Input: dimensioned drawing with shaded views. Units: mm. Origin: part minimum x, y, z. A direction names the side the tool comes from. Round coordinates to 2 decimals unless told otherwise and drop trailing zeros. Loops run counter-clockwise (first coordinate to the right, second up) from the corner with the lowest first, then second, coordinate; pieces in that order, holes last. Notation, with made-up numbers: (-16, 38.5) - (16, 38.5) arc R8 cw to (16, 43.5) - close; hole circle Ø6 at (31.5, 9.25). An arc over 180 degrees is marked (long way). One line per question, with ' | ' between items. Start each with the question number.
Item 1: Material intervals for line 1 along Z through (x, y) = (4.25, 13.75); line 2 along Z through (x, y) = (3, 7.25); line 3 along Y through (x, z) = (12.75, 0.6), sorted ascending.
Item 2: Section C-C, the plane y = 14.75. Return loops of the section in (x, z).
Item 3: First-contact query: pin 1 (1.4 mm diameter, centred on x = 11, z = 1, fed in from +Y); pin 2 (3 mm diameter, centred on y = 4.5, z = 4, fed in from +X); pin 3 (2.5 mm diameter, centred on x = 3.5, y = 12, fed in from -Z); pin 4 (1.4 mm diameter, centred on y = 11, z = 0.5, fed in from +X). Flat tips, straight axial feed; report the tip coordinate or a pass-through.
Item 4: Section B-B, the plane y = 10.5. Return loops of the section in (x, z), plus the area to 3 significant figures.
Item 5: Section A-A, the plane x = 12. Return loops of the section in (y, z).
Item 6: Draft query along Z for the marked faces 4, 5 and 6. Return one class per face: pulls with the +Z half, pulls with the -Z half, needs draft (parallel to the pull), parting line crosses it, or undercut.
Item 7: Set-up query: the marked faces 1, 2 and 3. Return all of +Z, -Z, +X, -X, +Y, -Y with unobstructed straight access to the full face (end or side cutting, diameter ignored); none if empty.
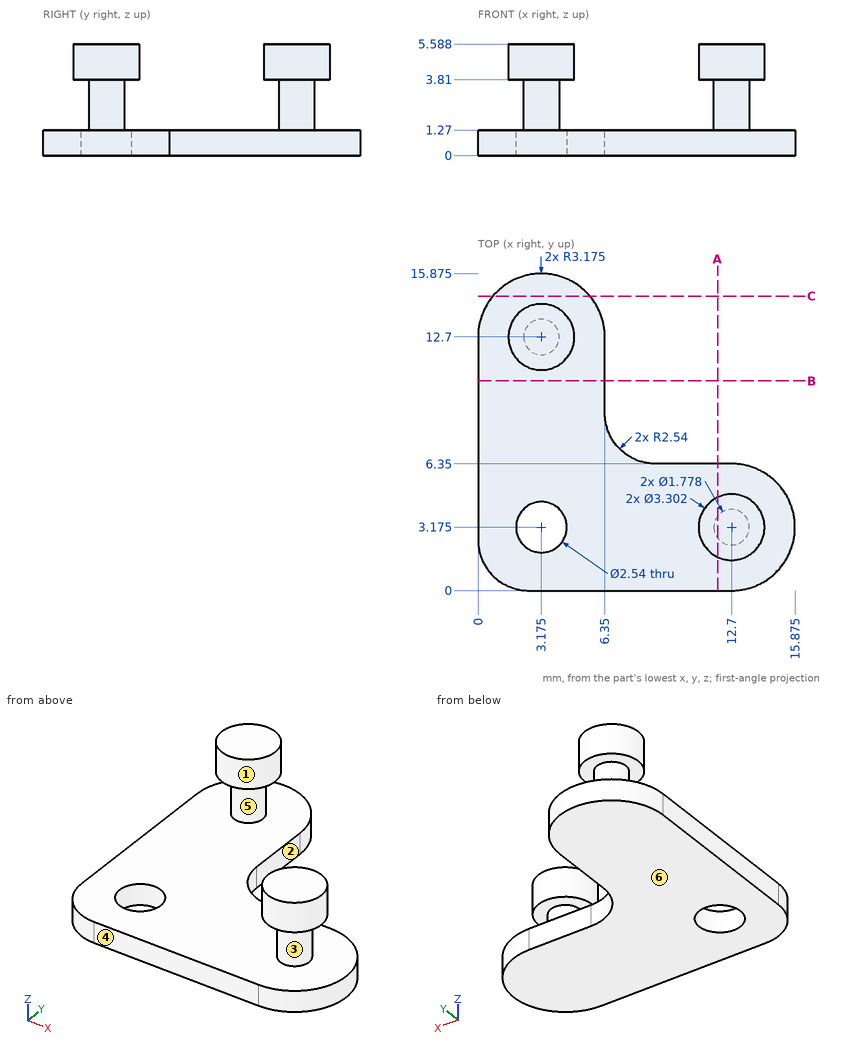
Return value:
1) line 1: 0 to 1.27, 3.81 to 5.59 | line 2: 0 to 1.27 | line 3: 0 to 6.35
2) outline: (0.75, 0) - (5.6, 0) - (5.6, 1.27) - (0.75, 1.27) - close
3) pin 1: y = 6.35 | pin 2: x = 14.35 | pin 3: z = 0 | pin 4: x = 6.35
4) outline: (0, 0) - (6.35, 0) - (6.35, 1.27) - (0, 1.27) - close | area: 8.06 mm2
5) outline: (0, 0) - (6.35, 0) - (6.35, 1.27) - (3.72, 1.27) - (3.72, 3.81) - (4.67, 3.81) - (4.67, 5.59) - (1.68, 5.59) - (1.68, 3.81) - (2.63, 3.81) - (2.63, 1.27) - (0, 1.27) - close
6) face 4: needs draft | face 5: undercut | face 6: pulls with the -Z half
7) face 1: +Z | face 2: +Z, -Z, +X, +Y | face 3: none
